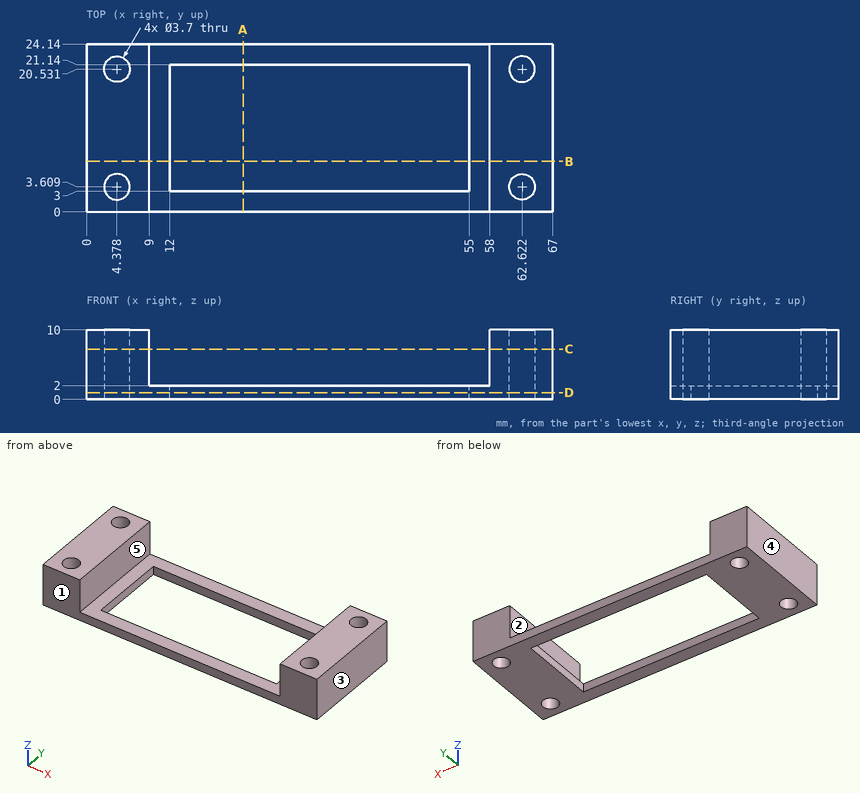
Design review of the part shown in the three views and the two pictorial views. Dimensions are in mm from the part's minimum x, y and z. A direction names the side the tool comes from. Give positions to 0.01 mm unless a question says otherwise; leave off trailing zeros. Loops run counter-clockwise (first coordinate to the right, second up) from the corner with the lowest first, then second, coordinate; pieces in that order, holes last. Notation, with made-up numbers: M 87.5,-19 L 134.5,-19 A15 ccw 134.5,-10 Z; hole C 89.5,-21.75 d5. An arc over 180 degrees is marked long. Answer as a JSON object with one key per item and string values.
Item 1: Machinability: for the marked faces 4 and 5, which of the approach directions +Z, -Z, +X, -X, +Y, -Y give a long, thin tool a straight path to every point of the face, cutting with its end or side? Answer none if there is none.
Output values:
{"face 4": "+Z, -Z, -X, +Y, -Y", "face 5": "+Z, +Y, -Y"}
Item 2: We need section C-C (z = 7.25). State the section outline as (x, y) points.
Output values:
{"outline": "M 0,0 L 9,0 L 9,24.14 L 0,24.14 Z; M 58,0 L 67,0 L 67,24.14 L 58,24.14 Z; hole C 4.38,3.61 d3.7; hole C 4.38,20.53 d3.7; hole C 62.62,3.61 d3.7; hole C 62.62,20.53 d3.7"}
Item 3: Mouldability with a two-part tool opening along X and no side actions: class the marked faces 1, 2 and 3 as pulls with the +X half, pulls with the -X half, needs draft (parallel to the pull), parting line crosses it, or undercut.
Output values:
{"face 1": "needs draft", "face 2": "undercut", "face 3": "pulls with the +X half"}
Item 4: We need section B-B (y = 7.25). State the section outline as (x, z) points.
Output values:
{"outline": "M 0,0 L 12,0 L 12,2 L 9,2 L 9,10 L 0,10 Z; M 55,0 L 67,0 L 67,10 L 58,10 L 58,2 L 55,2 Z"}
Item 5: We need section D-D (z = 1). State the section outline as (x, y) points.
Output values:
{"outline": "M 0,0 L 67,0 L 67,24.14 L 0,24.14 Z; hole C 4.38,3.61 d3.7; hole C 4.38,20.53 d3.7; hole M 12,3 L 55,3 L 55,21.14 L 12,21.14 Z; hole C 62.62,3.61 d3.7; hole C 62.62,20.53 d3.7"}
Item 6: Wall thickness on line 1 along X through (y, z) = (7, 5); line 2 along X through (y, z) = (19.25, 1) (1 decimal); line 3 along X through (y, z) = (4, 4.5) (1 decimal): over which ranges is each line inside the solid? List them lowest first.
Output values:
{"line 1": "x = 0 to 9, 58 to 67", "line 2": "x = 0 to 3, 5.7 to 12, 55 to 61.3, 64 to 67", "line 3": "x = 0 to 2.6, 6.2 to 9, 58 to 60.8, 64.4 to 67"}
Item 7: We need section A-A (x = 22.5). State the section outline as (y, z) points.
Output values:
{"outline": "M 0,0 L 3,0 L 3,2 L 0,2 Z; M 21.14,0 L 24.14,0 L 24.14,2 L 21.14,2 Z"}
Item 8: For P1, Ø5, axis at x = 38.5, y = 5, coming from the +Z side, flat-tipped, find the tip position at first contact; note if it passes through.
Output values:
{"P1": "stops at z = 2"}
